from build123d import *

# Parameters (mm, degrees)
F0_W      = 101.6
F0_H      = 152.4
F1_DEPTH  = 2.54
F2_W      = 12.7
F2_H      = 68.58
F3_DEPTH  = 2.541
F4_SIZE2  = 12.69999
F4_SIZE   = 12.69999
F5_R      = 12.446
F6_W      = 58.42
F6_H      = 12.7
F7_DEPTH  = 2.541
F8_W      = 12.7
F8_H      = 68.58
F9_DEPTH  = 2.541
F10_R     = 12.69999
F11_SIZE2 = 12.69999
F11_SIZE  = 12.69999
F12_W     = 12.7
F12_H     = 68.58
F13_DEPTH = 2.541
F14_SIZE2 = 12.69999
F14_SIZE  = 12.69999
F15_R     = 12.69999
F16_W     = 12.7
F16_H     = 68.58
F17_DEPTH = 2.541
F18_SIZE2 = 12.69999
F18_SIZE  = 12.69999
F19_R     = 12.69999
F20_W     = 58.42
F20_H     = 12.7
F21_DEPTH = 2.541
F23_DEPTH = 25.4
F25_DEPTH = 25.4
F27_DEPTH = 25.4
F28_W     = 2.54
F28_H     = 10.16
F29_DEPTH = 25.4
F30_W     = 2.54
F30_H     = 10.16
F31_DEPTH = 25.4
F32_W     = 15.24
F32_H     = 2.54
F33_DEPTH = 25.4


# Not quite as in the source:
# - a fillet or chamfer is up to 0.001 mm smaller than in the source, because OpenCascade refuses the exact size


with BuildPart() as f1:
    # F0 (on Top) → F1 (new body)
    with BuildSketch(Plane.XY):
        Rectangle(F0_W, F0_H)
    extrude(amount=F1_DEPTH)

    # F2 (on face) → F3 (cut, through all)
    with BuildSketch(Plane.XY.offset(2.54)):
        with Locations((-38.1, 35.56)):
            Rectangle(F2_W, F2_H)
    extrude(amount=-F3_DEPTH, mode=Mode.SUBTRACT)

    # F4 (size 12.7 and 12.7 in the source; OpenCascade refuses exactly that, so slightly less here)
    f4_edges = [f1.edges().sort_by_distance(p)[0] for p in [
        (-31.75, 1.27, 1.27),
    ]]
    chamfer(f4_edges, length=F4_SIZE, length2=F4_SIZE2)

    # F5
    f5_edges = [f1.edges().sort_by_distance(p)[0] for p in [
        (-44.45, 69.85, 1.27),
    ]]
    fillet(f5_edges, radius=F5_R)

    # F6 (on face) → F7 (cut, through all)
    with BuildSketch(Plane.XY.offset(2.54)):
        with Locations((0, 63.5)):
            Rectangle(F6_W, F6_H)
    extrude(amount=-F7_DEPTH, mode=Mode.SUBTRACT)

    # F8 (on face) → F9 (cut, through all)
    with BuildSketch(Plane.XY.offset(2.54)):
        with Locations((38.1, 35.56)):
            Rectangle(F8_W, F8_H)
    extrude(amount=-F9_DEPTH, mode=Mode.SUBTRACT)

    # F10 (radius 12.7 in the source; OpenCascade refuses exactly that, so slightly less here)
    f10_edges = [f1.edges().sort_by_distance(p)[0] for p in [
        (44.45, 69.85, 1.27),
    ]]
    fillet(f10_edges, radius=F10_R)

    # F11 (size 12.7 and 12.7 in the source; OpenCascade refuses exactly that, so slightly less here)
    f11_edges = [f1.edges().sort_by_distance(p)[0] for p in [
        (31.75, 1.27, 1.27),
    ]]
    chamfer(f11_edges, length=F11_SIZE, length2=F11_SIZE2)

    # F12 (on face) → F13 (cut, through all)
    with BuildSketch(Plane.XY.offset(2.54)):
        with Locations((-38.1, -35.56)):
            Rectangle(F12_W, F12_H)
    extrude(amount=-F13_DEPTH, mode=Mode.SUBTRACT)

    # F14 (size 12.7 and 12.7 in the source; OpenCascade refuses exactly that, so slightly less here)
    f14_edges = [f1.edges().sort_by_distance(p)[0] for p in [
        (-31.75, -1.27, 1.27),
    ]]
    chamfer(f14_edges, length=F14_SIZE, length2=F14_SIZE2)

    # F15 (radius 12.7 in the source; OpenCascade refuses exactly that, so slightly less here)
    f15_edges = [f1.edges().sort_by_distance(p)[0] for p in [
        (-44.45, -69.85, 1.27),
    ]]
    fillet(f15_edges, radius=F15_R)

    # F16 (on face) → F17 (cut, through all)
    with BuildSketch(Plane.XY.offset(2.54)):
        with Locations((38.1, -35.56)):
            Rectangle(F16_W, F16_H)
    extrude(amount=-F17_DEPTH, mode=Mode.SUBTRACT)

    # F18 (size 12.7 and 12.7 in the source; OpenCascade refuses exactly that, so slightly less here)
    f18_edges = [f1.edges().sort_by_distance(p)[0] for p in [
        (31.75, -1.27, 1.27),
    ]]
    chamfer(f18_edges, length=F18_SIZE, length2=F18_SIZE2)

    # F19 (radius 12.7 in the source; OpenCascade refuses exactly that, so slightly less here)
    f19_edges = [f1.edges().sort_by_distance(p)[0] for p in [
        (44.45, -69.85, 1.27),
    ]]
    fillet(f19_edges, radius=F19_R)

    # F20 (on face) → F21 (cut, through all)
    with BuildSketch(Plane.XY.offset(2.54)):
        with Locations((0, -63.5)):
            Rectangle(F20_W, F20_H)
    extrude(amount=-F21_DEPTH, mode=Mode.SUBTRACT)

    # F22 (on face) → F23 (cut)
    with BuildSketch(Plane.XY.offset(2.54)):
        Polygon((-31.75, 6.35), (-42.2502954744, 0), (-31.75, -6.35), (31.75, -6.35), (42.2502954744, 0), (31.75, 6.35), align=None)
    extrude(amount=-F23_DEPTH, mode=Mode.SUBTRACT)

    # F24 (on face) → F25 (cut)
    with BuildSketch(Plane.XY.offset(2.54)):
        Polygon((-50.8, -76.2), (-39.37, -76.2), (-41.91, -73.66), (-50.8, -73.66), align=None)
        Polygon((41.91, -73.66), (39.37, -76.2), (50.8, -76.2), (50.8, -73.66), align=None)
    extrude(amount=-F25_DEPTH, mode=Mode.SUBTRACT)

    # F26 (on face) → F27 (cut)
    with BuildSketch(Plane.XY.offset(2.54)):
        Polygon((-39.37, 76.2), (-50.8, 76.2), (-50.8, 73.66), (-41.91, 73.66), align=None)
        Polygon((50.8, 76.2), (39.37, 76.2), (41.91, 73.66), (50.8, 73.66), align=None)
    extrude(amount=-F27_DEPTH, mode=Mode.SUBTRACT)

    # F28 (on face) → F29 (cut)
    with BuildSketch(Plane.XY.offset(2.54)):
        with Locations((49.53, 36.83)):
            Rectangle(F28_W, F28_H)
        with Locations((49.53, -36.83)):
            Rectangle(F28_W, F28_H)
    extrude(amount=-F29_DEPTH, mode=Mode.SUBTRACT)

    # F30 (on face) → F31 (cut)
    with BuildSketch(Plane.XY.offset(2.54)):
        with Locations((-49.53, 36.83)):
            Rectangle(F30_W, F30_H)
        with Locations((-49.53, -36.83)):
            Rectangle(F30_W, F30_H)
    extrude(amount=-F31_DEPTH, mode=Mode.SUBTRACT)

    # F32 (on face) → F33 (cut)
    with BuildSketch(Plane.XY.offset(2.54)):
        with Locations((-43.18, -74.93)):
            Rectangle(F32_W, F32_H)
        with Locations((43.18, -74.93)):
            Rectangle(F32_W, F32_H)
        with Locations((-43.18, 74.93)):
            Rectangle(F32_W, F32_H)
        with Locations((43.18, 74.93)):
            Rectangle(F32_W, F32_H)
    extrude(amount=-F33_DEPTH, mode=Mode.SUBTRACT)


solid = f1.part
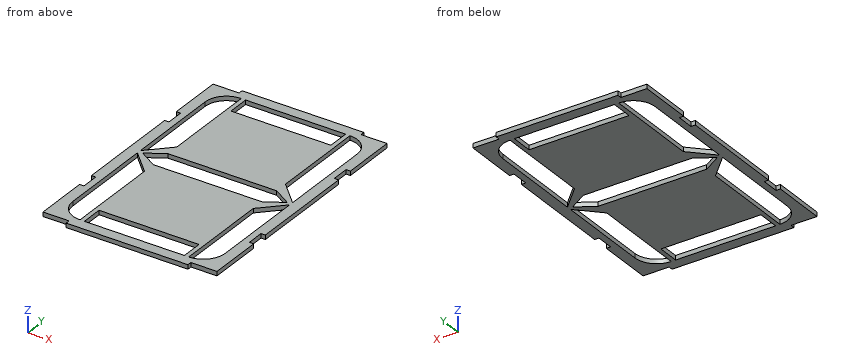
Read the model definition and answer for the solid it produces. Units are mm, in the model's axes. Coordinates: 2 decimals unless noted, no trailing zeros. Order: outer loops, then holes, each group sorted by start corner. A loop starts at its lowest first (then second) coordinate and runs counter-clockwise, first axis right, second up. Notation, with made-up numbers: (51.5, -19.75) -> (86.5, -19.75) arc R8 ccw to (86.5, -15.75) -> close; hole circle Ø3 at (46.5, -39). An arc over 180 degrees is marked (long way). Answer as a JSON object with one key per item and string values.
1) A cutting plane is placed at A-A, the plane y = -34. Determine the outline of the cut face in (x, z), plus the area to 3 significant figures.
Model answer:
{"outline": "(-48.26, 0) -> (-44.45, 0) -> (-44.45, 2.54) -> (-48.26, 2.54) -> close; (-31.75, 0) -> (31.75, 0) -> (31.75, 2.54) -> (-31.75, 2.54) -> close; (44.45, 0) -> (48.26, 0) -> (48.26, 2.54) -> (44.45, 2.54) -> close", "area": "181 mm²"}
2) A cutting plane is placed at C-C, the plane z = 1.75. State how many separate pieces and enclosed holes the cut face has, plus the area to 3 significant figures.
Model answer:
{"separate pieces": "1", "enclosed holes": "7", "area": "9,780 mm²"}
3) A cutting plane is placed at B-B, the plane x = 21. Determine the outline of the cut face in (y, z).
Model answer:
{"outline": "(-76.2, 0) -> (-69.85, 0) -> (-69.85, 2.54) -> (-76.2, 2.54) -> close; (-57.15, 0) -> (-6.35, 0) -> (-6.35, 2.54) -> (-57.15, 2.54) -> close; (6.35, 0) -> (57.15, 0) -> (57.15, 2.54) -> (6.35, 2.54) -> close; (69.85, 0) -> (76.2, 0) -> (76.2, 2.54) -> (69.85, 2.54) -> close"}
4) A cutting plane is placed at D-D, the plane y = 24. Determine the outline of the cut face in (x, z), plus the area to 3 significant figures.
Model answer:
{"outline": "(-50.8, 0) -> (-44.45, 0) -> (-44.45, 2.54) -> (-50.8, 2.54) -> close; (-31.75, 0) -> (31.75, 0) -> (31.75, 2.54) -> (-31.75, 2.54) -> close; (44.45, 0) -> (50.8, 0) -> (50.8, 2.54) -> (44.45, 2.54) -> close", "area": "194 mm²"}
5) Consider line 1 along X through (y, z) = (46, 2.35); line 2 along Y through (x, z) = (-13.5, 2.4); line 3 along X through (y, z) = (-34, 0.7). Determine where each line is inside the solid, lowest interval first. Write a range as from..to.
Model answer:
{"line 1": "x = -50.8..-44.45, -31.75..31.75, 44.45..50.8", "line 2": "y = -76.2..-69.85, -57.15..-6.35, 6.35..57.15, 69.85..76.2", "line 3": "x = -48.26..-44.45, -31.75..31.75, 44.45..48.26"}
6) Each of these flat-tipped pins is pushed along its axis until it touches: pin 1 (1.3 mm diameter, centred on y = 75, z = 1.5, fed in from -X); pin 2 (0.8 mm diameter, centred on x = -49.5, z = 2, fed in from +Y). Where does it stop, or does it pass through?
Model answer:
{"pin 1": "stops at x = -35.56", "pin 2": "stops at y = 73.66"}
